```python
from build123d import *

# Parameters (mm, degrees)
SKETCH1_R           = 4.05
BOSS_EXTRUDE1_DEPTH = 20
BOSS_EXTRUDE2_DEPTH = 5
SKETCH3_R           = 4.75
SKETCH3_R_2         = 4.05
BOSS_EXTRUDE3_DEPTH = 7
CHAMFER1_SIZE       = 0.5
SKETCH4_R           = 1.3
CUT_EXTRUDE1_DEPTH  = 10.5


with BuildPart() as part:
    # Sketch1 → Boss-Extrude1 (new body)
    with BuildSketch(Plane(origin=(0, 0, 0), x_dir=(1, 0, 0), z_dir=(0, 1, 0))):
        Circle(SKETCH1_R)
        Polygon((1.187868906, 2.047510878), (-1.179261982, 2.052480088), (-2.367130888, 0.00496921), (-1.187868906, -2.047510878), (1.179261982, -2.052480088), (2.367130888, -0.00496921), align=None, mode=Mode.SUBTRACT)
    extrude(amount=BOSS_EXTRUDE1_DEPTH)

    # Sketch2 → Boss-Extrude2 (add)
    with BuildSketch(Plane.XZ):
        Polygon((1.187868906, -2.047510878), (2.367130888, 0.00496921), (1.179261982, 2.052480088), (-1.187868906, 2.047510878), (-2.367130888, -0.00496921), (-1.179261982, -2.052480088), align=None)
    extrude(amount=-BOSS_EXTRUDE2_DEPTH)

    # Sketch3 → Boss-Extrude3 (add)
    with BuildSketch(Plane(origin=(0, 13, 0), x_dir=(-1, 0, 0), z_dir=(0, -1, 0))):
        Circle(SKETCH3_R)
        Circle(SKETCH3_R_2, mode=Mode.SUBTRACT)
    extrude(amount=-BOSS_EXTRUDE3_DEPTH)

    # Chamfer1
    chamfer1_edges = [part.edges().sort_by_distance(p)[0] for p in [
        (1.777499897, 20, -1.021270834),
        (0.004303462, 20, -2.049995483),
        (-1.773196435, 20, -1.028724649),
        (-1.777499897, 20, 1.021270834),
        (-0.004303462, 20, 2.049995483),
        (1.773196435, 20, 1.028724649),
    ]]
    chamfer(chamfer1_edges, length=CHAMFER1_SIZE)

    # Sketch4 → Cut-Extrude1 (cut, through all)
    with BuildSketch(Plane(origin=(0, 0, -4.75), x_dir=(-1, 0, 0), z_dir=(0, 0, -1))):
        with Locations((0, 16.319152566)):
            Circle(SKETCH4_R)
    extrude(amount=-CUT_EXTRUDE1_DEPTH, mode=Mode.SUBTRACT)


solid = part.part
```
Read the model definition and answer for the solid it produces. Units are mm, in the model's axes. A direction names the side the tool comes from. Give positions to 0.01 mm unless a question says otherwise; leave off trailing zeros. Order: outer loops, then holes, each group sorted by start corner. A loop starts at its lowest first (then second) coordinate and runs counter-clockwise, first axis right, second up. Notation, with made-up numbers: (9, -20) -> (35, -20) arc R6 ccw to (35, -15) -> close; hole circle Ø5 at (-29, -39.5). An arc over 180 degrees is marked (long way). One line per item, written item: value. Start each with the question number.
(1) The part is cut by section C-C (z = 1). Determine the outline of the cut face in (x, y), and give its area (3 significant figures).
(2) The part is cut by section D-D (x = -2.75). Determine the outline of the cut face in (y, z), and give its area (3 significant figures).
(3) For a pull along X with two mould halves and no side action, classify faces 3 (the flat face through (-2.002, 19.746, 1.126)), 4 (the flat face through (2, 13, -4)), 5 (the cylindrical face through (-0.878, 6.409, 3.954)) as released by +X, released by -X, zero draft, split by the parting line, or undercut.
(4) Straight lines are drawn through the part: L1, parallel to Z at x = 1, y = 17.75; L2, parallel to Y at x = 0, z = 3.4; L3, parallel to Y at x = 0.75, z = -2. For each, find the intervals that lie inside material, in ascending order.
(5) The part is cut by section A-A (y = 13.5). Determine the outline of the cut face in (x, z), and give its area (3 significant figures).
(6) The part is cut by section B-B (x = 0). Determine the outline of the cut face in (y, z), and give its area (3 significant figures).
(7) Flat-ended cylindrical pins translate along their axes: P1, Ø3, axis at x = 0, y = 16.32, coming from the -Z side; P2, Ø4, axis at y = 10, z = 1, coming from the -X side; P3, Ø2, axis at x = -0.5, z = 0, coming from the +Y side. Find the tip coordinate at first contact, or state that the pin passes through.
(8) A tool of negligible diameter and unlimited length cuts with its end or side. For faces 1 (the flat face through (-1.786, 12.148, 1.007)), 2 (the flat face through (0, 0, 0)), from which of +Z, -Z, +X, -X, +Y, -Y can it reach the whole face along a straight path? Write none if from no direction.
Taken from the geometry:
1. outline: (-4.64, 13) -> (-3.92, 13) -> (-3.92, 0) -> (3.92, 0) -> (3.92, 13) -> (4.64, 13) -> (4.64, 20) -> (2.37, 20) -> (1.79, 19.5) -> (1.79, 5) -> (-1.79, 5) -> (-1.79, 19.5) -> (-2.37, 20) -> (-4.64, 20) -> close
1. area: 113 mm^2
2. outline: (0, -2.97) -> (13, -2.97) -> (13, -3.87) -> (20, -3.87) -> (20, -0.34) -> (19.83, -0.01) -> (20, 0.33) -> (20, 3.87) -> (13, 3.87) -> (13, 2.97) -> (0, 2.97) -> close
2. area: 131 mm^2
3. face 3: undercut
3. face 4: zero draft
3. face 5: split by the parting line
4. L1: -4.64 to -2.05, 2.05 to 4.64
4. L2: 0 to 15.02, 17.62 to 20
4. L3: 0 to 5
5. outline: circle Ø9.5 at (0, 0); hole (-2.37, 0) -> (-1.18, -2.05) -> (1.19, -2.05) -> (2.37, 0) -> (1.18, 2.05) -> (-1.19, 2.05) -> close
5. area: 56.3 mm^2
6. outline: (0, -4.05) -> (13, -4.05) -> (13, -4.75) -> (15.02, -4.75) -> (15.02, -2.05) -> (5, -2.05) -> (5, 2.05) -> (15.02, 2.05) -> (15.02, 4.75) -> (13, 4.75) -> (13, 4.05) -> (0, 4.05) -> close; (17.62, -4.75) -> (20, -4.75) -> (20, -2.55) -> (19.5, -2.05) -> (17.62, -2.05) -> close; (17.62, 2.05) -> (19.5, 2.05) -> (20, 2.55) -> (20, 4.75) -> (17.62, 4.75) -> close
6. area: 96.0 mm^2
7. P1: z = -4.75
7. P2: x = -4.05
7. P3: y = 5
8. face 1: +Y
8. face 2: +Z, -Z, +X, -X, -Y
